from build123d import *

# Parameters (mm, degrees)
SKETCH4_R           = 42.545
BOSS_EXTRUDE2_DEPTH = 1
SKETCH5_R           = 29.845
CUT_EXTRUDE5_DEPTH  = 2
SKETCH6_R           = 3.175
CUT_EXTRUDE6_DEPTH  = 2
CIRPATTERN1_COUNT   = 8
CUT_EXTRUDE11_DEPTH = 2


with BuildPart() as part:
    # Sketch4 → Boss-Extrude2 (new body)
    with BuildSketch(Plane.XY):
        Circle(SKETCH4_R)
    extrude(amount=BOSS_EXTRUDE2_DEPTH)

    # Sketch5 → Cut-Extrude5 (cut, through all)
    with BuildSketch(Plane.XY.offset(1)):
        Circle(SKETCH5_R)
    extrude(amount=-CUT_EXTRUDE5_DEPTH, mode=Mode.SUBTRACT)

    # Sketch6 → Cut-Extrude6 (cut, through all)
    with BuildSketch(Plane.XY.offset(1)):
        with Locations((36.195, 0)):
            Circle(SKETCH6_R)
    cut_extrude6 = extrude(amount=-CUT_EXTRUDE6_DEPTH, mode=Mode.SUBTRACT)

    # CirPattern1: Cut-Extrude6 ×8 about axis
    cirpattern1_axis = Axis((0, 0, 0), (0, 0, 1))
    for i in range(1, CIRPATTERN1_COUNT):
        add(cut_extrude6.rotate(cirpattern1_axis, i * 360 / CIRPATTERN1_COUNT), mode=Mode.SUBTRACT)

    # Sketch8 → Cut-Extrude11 (cut, through all)
    with BuildSketch(Plane.XY.offset(1)):
        Polygon((42.34042777, 18.912617514), (23.56719567, 11.136490168), (24.539211588, 8.789836155), (43.312443689, 16.565963501), align=None)
        Polygon((17.697597616, 39.407110255), (15.350943603, 40.379126173), (14.864935644, 39.205799167), (17.211589657, 38.233783248), align=None)
        Polygon((-15.350943603, 40.379126173), (-17.697597616, 39.407110255), (-17.211589657, 38.233783248), (-14.864935644, 39.205799167), align=None)
        Polygon((-39.407110255, 17.697597616), (-40.379126173, 15.350943603), (-39.205799167, 14.864935644), (-38.233783248, 17.211589657), align=None)
        Polygon((-40.379126173, -15.350943603), (-39.407110255, -17.697597616), (-38.233783248, -17.211589657), (-39.205799167, -14.864935644), align=None)
        Polygon((-17.697597616, -39.407110255), (-15.350943603, -40.379126173), (-14.864935644, -39.205799167), (-17.211589657, -38.233783248), align=None)
        Polygon((15.350943603, -40.379126173), (17.697597616, -39.407110255), (17.211589657, -38.233783248), (14.864935644, -39.205799167), align=None)
        Polygon((39.407110255, -17.697597616), (40.379126173, -15.350943603), (39.205799167, -14.864935644), (38.233783248, -17.211589657), align=None)
    extrude(amount=-CUT_EXTRUDE11_DEPTH, mode=Mode.SUBTRACT)


solid = part.part
Work out the finished part from the listing and answer in its coordinate system (mm). A direction names the side the tool comes from. Round coordinates to 2 decimals unless told otherwise and drop trailing zeros. Write each loop counter-clockwise with the first axis right and the second up, starting at its lowest first coordinate (ties: lowest second). Pieces come first, ordered by that corner, then holes. Notation, with made-up numbers: (-15, 76) -> (31, 76) arc R25 cw to (31, 111) -> close; hole circle Ø7 at (2, 23). An arc over 180 degrees is marked (long way). Write each question's results on one line, items separated by ' | '.
Item 1: A cutting plane is placed at A-A, the plane y = 0. Determine the outline of the cut face in (x, z) (3 decimals), plus the area to 3 significant figures.
Result set:
outline: (-42.545, 0) -> (-39.37, 0) -> (-39.37, 1) -> (-42.545, 1) -> close; (-33.02, 0) -> (-29.845, 0) -> (-29.845, 1) -> (-33.02, 1) -> close; (29.845, 0) -> (33.02, 0) -> (33.02, 1) -> (29.845, 1) -> close; (39.37, 0) -> (42.545, 0) -> (42.545, 1) -> (39.37, 1) -> close | area: 12.7 mm^2
Item 2: A cutting plane is placed at C-C, the plane x = -35. Determine the outline of the cut face in (y, z), plus the area to 3 significant figures.
Result set:
outline: (-24.19, 0) -> (-2.94, 0) -> (-2.94, 1) -> (-24.19, 1) -> close; (2.94, 0) -> (24.19, 0) -> (24.19, 1) -> (2.94, 1) -> close | area: 42.5 mm^2
Item 3: A flat-ended cylindrical pin translates along its axis: P1, Ø2, axis at x = 33, y = -11, coming from the -Z side. Find the tip coordinate at first contact, or state that the pin passes through.
Result set:
P1: z = 0
Item 4: The mould has two halves that part along Y. Classify faces 3 (the face through (-29.931, 30.236, 0.493)), 4 (the face through (0.954, -39.223, 0.507)), 5 (the face through (42.544, -0.216, 0.493)): +Y half, -Y half, draft (parallel to the pull), parting line (faces both ways), or undercut.
Result set:
face 3: +Y half | face 4: undercut | face 5: parting line
Item 5: Which of the six approach directions +Z, -Z, +X, -X, +Y, -Y give full straight-line access (tool end or side, diameter ignored) to faces 1 (the face through (29.931, -30.236, 0.493)), 2 (the face through (33.822, 12.635, 0.507))?
Result set:
face 1: +Z, -Z, +X, -Y | face 2: +Z, -Z
Item 6: Find the intervals of material crossed by line 1 along Y through (x, z) = (34.5, 0.9) (3 decimals); line 2 along Y through (x, z) = (-16, 0.85); line 3 along Y through (x, z) = (-13, 0.3), in increasing order. Write a range as [from, to].
Result set:
line 1: [-24.896, -2.685], [2.685, 12.916], [15.665, 24.896] | line 2: [-38.74, -25.19], [25.19, 38.74] | line 3: [-40.51, -26.86], [26.86, 40.51]
Item 7: A cutting plane is placed at D-D, the plane x = 19. Determine the outline of the cut face in (y, z), plus the area to 3 significant figures.
Result set:
outline: (-38.07, 0) -> (-23.02, 0) -> (-23.02, 1) -> (-38.07, 1) -> close; (23.02, 0) -> (38.07, 0) -> (38.07, 1) -> (23.02, 1) -> close | area: 30.1 mm^2
